```python
from build123d import *

# Parameters (mm, degrees)
ESQUISSE1_R             = 10
ESQUISSE1_R_2           = 6
BOSS_EXTRU_1_DEPTH      = 35
ESQUISSE2_W             = 4
ESQUISSE2_H             = 6.064626471
ENL_V_MAT_EXTRU_1_DEPTH = 38.749172176
CHANFREIN1_SIZE         = 0.5


with BuildPart() as part:
    # Esquisse1 → Boss.-Extru.1 (new body)
    with BuildSketch(Plane(origin=(0, 0, 0), x_dir=(0, 0, -1), z_dir=(1, 0, 0))):
        Circle(ESQUISSE1_R)
        Circle(ESQUISSE1_R_2, mode=Mode.SUBTRACT)
    extrude(amount=BOSS_EXTRU_1_DEPTH)

    # Esquisse2 → Enlèv. mat.-Extru.1 (cut, through all)
    with BuildSketch(Plane.ZY):
        with Locations((0, 4.767686765)):
            Rectangle(ESQUISSE2_W, ESQUISSE2_H)
    extrude(amount=-ENL_V_MAT_EXTRU_1_DEPTH, mode=Mode.SUBTRACT)

    # Chanfrein1
    chanfrein1_edges = [part.edges().sort_by_distance(p)[0] for p in [
        (0, 0, 10),
        (35, 0, 10),
    ]]
    chamfer(chanfrein1_edges, length=CHANFREIN1_SIZE)


solid = part.part
```
Verification items for the finished model (mm, model axes). A direction names the side the tool comes from. Give positions to 0.01 mm unless a question says otherwise; leave off trailing zeros. Loops run counter-clockwise (first coordinate to the right, second up) from the corner with the lowest first, then second, coordinate; pieces in that order, holes last. Notation, with made-up numbers: M 77,15 L 89,15 A28 ccw 89,44 Z; hole C 55,84.25 d7. An arc over 180 degrees is marked long. Return JSON: item names as keys, results as strings.
1) Gauge pin test, flat ends, axial feed: P1, Ø1, axis at x = 26, z = 3.5, coming from the +Y side; P2, Ø2.5, axis at x = 12, y = 7, coming from the +Z side; P3, Ø3, axis at y = 2, z = 2, coming from the +X side; P4, Ø5, axis at x = 25.5, z = -7.5, coming from the +Y side. Record the tip position at first contact, or that the pin passes through.
Findings:
{"P1": "stops at y = 9.54", "P2": "stops at z = 8.18", "P3": "passes through", "P4": "stops at y = 8.66"}
2) Mould release check, pull along Z, two halves, no side actions. Record for faces 1 (the flat face through (17, 7, 2)), 2 (the flat face through (35, -6.2, 0.1)), 3 (the cylindrical face through (17.26, -9.76, 2.17)), 4 (the flat face through (17, 7.8, 0)): released by +Z, released by -Z, zero draft, split by the parting line, or undercut.
Findings:
{"face 1": "undercut", "face 2": "zero draft", "face 3": "split by the parting line", "face 4": "undercut"}
3) Section check A-A, the plane y = 0. Enter the section's corners in (x, z), and give its area (4 significant figures).
Findings:
{"outline": "M 0,-9.5 L 0.5,-10 L 34.5,-10 L 35,-9.5 L 35,-6 L 0,-6 Z; M 0,6 L 35,6 L 35,9.5 L 34.5,10 L 0.5,10 L 0,9.5 Z", "area": "279.5 mm2"}
4) Section check B-B, the plane z = 0. Enter the section's corners in (x, y), and give its area (4 significant figures).
Findings:
{"outline": "M 0,-9.5 L 0.5,-10 L 34.5,-10 L 35,-9.5 L 35,-6 L 0,-6 Z; M 0,7.8 L 35,7.8 L 35,9.5 L 34.5,10 L 0.5,10 L 0,9.5 Z", "area": "216.5 mm2"}
5) Section check C-C, the plane x = 30.5. Enter the section's corners in (y, z).
Findings:
{"outline": "C 0,0 d20; hole M 5.66,-2 L 7.8,-2 L 7.8,2 L 5.66,2 A6 ccw long Z"}
6) Material ranges on L1, parallel to Y at x = 20.5, z = 0; L2, parallel to Y at x = 6.5, z = -1.75; L3, parallel to Z at x = 7, y = 7, recorded low to high. Write a range as [from, to].
Findings:
{"L1": "y = [-10, -6], [7.8, 10]", "L2": "y = [-9.85, -5.74], [7.8, 9.85]", "L3": "z = [-7.14, -2], [2, 7.14]"}
7) Tool access check on faces 5 (the flat face through (0, -6.2, 0.1)), 6 (the flat face through (17, 7, -2)). Record the directions out of +Z, -Z, +X, -X, +Y, -Y that give a thin tool (end or side, any length) a straight path to the whole face; none if there is none.
Findings:
{"face 5": "+Z, -Z, -X, +Y, -Y", "face 6": "+X, -X"}
